Build history of the part. All positions in model axes, mm. Round coordinates to 2 decimals unless told otherwise and drop trailing zeros. Loops run counter-clockwise (first coordinate to the right, second up) from the corner with the lowest first, then second, coordinate; pieces in that order, holes last. Notation, with made-up numbers: (60, -28) - (103, -28) arc R24 ccw to (103, 10) - close; hole circle Ø10 at (7.5, -9). An arc over 180 degrees is marked (long way). Use a Markdown table: item, result.
Autodesk Inventor part; units mm, degrees
ref_plane "YZ Plane" through (0, 0, 0) normal (1, 0, 0) x (0, 1, 0)
ref_plane "XZ Plane" through (0, 0, 0) normal (0, 1, 0) x (-1, 0, 0)
ref_plane "XY Plane" through (0, 0, 0) normal (0, 0, 1) x (1, 0, 0)
sketch "Sketch1" plane through (0, 0, 0) normal (0, 0, 1) x (1, 0, 0)
  circle A0 centre (-0.2682, 25.3986) radius 2.0955
  circle A1 centre (0, 0) radius 5.2
  line L0 (-19.0905, 68.1502) -> (-19.0905, 45.2902)
  line L1 (-22.4814, 68.1502) -> (-22.4814, 45.2902)
  line L2 (28.3186, 68.1502) -> (28.3186, 45.2902)
  line L3 (31.7095, 68.1502) -> (31.7095, 45.2902)
  arc A2 (-19.0905, 68.1502) -> (-22.4814, 68.1502) centre (-20.7859, 68.1502) ccw
  arc A3 (-22.4814, 45.2902) -> (-19.0905, 45.2902) centre (-20.7859, 45.2902) ccw
  arc A4 (31.7095, 68.1502) -> (28.3186, 68.1502) centre (30.0141, 68.1502) ccw
  arc A5 (28.3186, 45.2902) -> (31.7095, 45.2902) centre (30.0141, 45.2902) ccw
  line L4 (-22.4814, 56.7202) -> (-30.1014, 56.7202)
  line L5 (-30.1014, 56.7202) -> (-30.1014, 73.8652)
  line L6 (31.7095, 56.7202) -> (39.3295, 56.7202)
  line L7 (39.3295, 56.7202) -> (39.3295, 73.8652)
  line L8 (36.1545, 77.0402) -> (-26.9264, 77.0402)
  line L9 (-30.1014, 56.7202) -> (-30.1014, 37.3371)
  line L10 (39.3295, 56.7202) -> (39.3295, 37.5617)
  line L11 (0, 0) -> (0, -10.16)
  line L12 (-2.3266, -6.5613) -> (-29.5927, 35.6134)
  line L13 (2.7652, -6.8864) -> (38.58, 35.5129)
  arc A6 (-30.1014, 37.3371) -> (-29.5927, 35.6134) centre (-26.9264, 37.3371) ccw
  arc A7 (-26.9264, 77.0402) -> (-30.1014, 73.8652) centre (-26.9264, 73.8652) ccw
  arc A8 (39.3295, 73.8652) -> (36.1545, 77.0402) centre (36.1545, 73.8652) ccw
  arc A9 (38.58, 35.5129) -> (39.3295, 37.5617) centre (36.1545, 37.5617) ccw
  arc A10 (-2.3266, -6.5613) -> (2.7652, -6.8864) centre (0.3398, -4.8376) ccw
  circle A11 centre (-8.0859, 47.3249) radius 2.1844
  circle A12 centre (17.3141, 47.3249) radius 2.1844
  point P0 (0, 0)
  point P1 (-30.1014, 77.0402)
  point P2 (-30.1014, 36.4002)
  point P3 (39.3295, 36.4002)
  dimension "d5" = 7.62
  dimension "d6" = 20.32
  dimension "d7" = 7.62
  dimension "d8" = 20.32
  dimension "d9" = 20.32
  dimension "d10" = 10.16
  dimension "d11" = 3.175
  dimension "d12" = 4.191
extrude "Extrusion1" add sketch "Sketch1" along normal blind 1.524
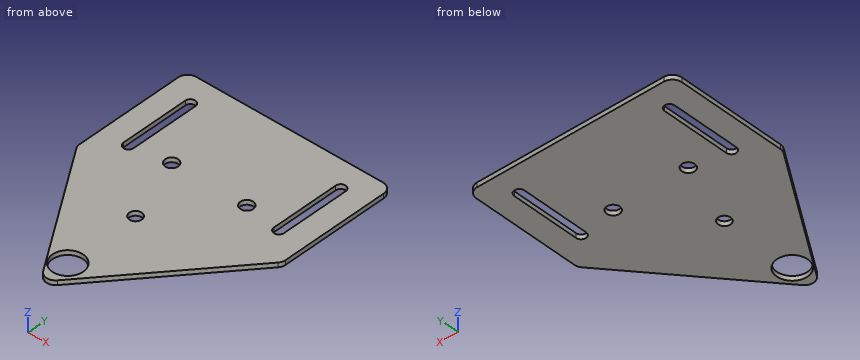
Q1. Cut at C-C, the plane x = 0. List the corners of the cut face in (y, z), plus the area to 3 significant figures.
Results found:
| item | result |
|---|---|
| outline | (-7.99, 0) - (-5.2, 0) - (-5.2, 1.52) - (-7.99, 1.52) - close; (5.2, 0) - (23.32, 0) - (23.32, 1.52) - (5.2, 1.52) - close; (27.48, 0) - (77.04, 0) - (77.04, 1.52) - (27.48, 1.52) - close |
| area | 107 mm2 |
Q2. Probe line 1 (X direction, y = 62, z = 0.9); line 2 (Y direction, x = 0, z = 0.6); line 3 (Y direction, x = 1, z = 1.2). List the from-to ranges inside material, lowest first.
Results found:
| item | result |
|---|---|
| line 1 | x = -30.1 to -22.48, -19.09 to 28.32, 31.71 to 39.33 |
| line 2 | y = -7.99 to -5.2, 5.2 to 23.32, 27.48 to 77.04 |
| line 3 | y = -7.94 to -5.1, 5.1 to 23.73, 27.07 to 77.04 |
Q3. Drop a flat-ended pin along its axis: pin 1 (4 mm diameter, centred on x = -0.27, y = 25.4, fed in from +Z). Give the stop position or say it passes through.
Results found:
| item | result |
|---|---|
| pin 1 | passes through |
Q4. Cut at D-D, the plane y = 0. List the corners of the cut face in (x, z), plus the area to 3 significant figures.
Results found:
| item | result |
|---|---|
| outline | (-6.57, 0) - (-5.2, 0) - (-5.2, 1.52) - (-6.57, 1.52) - close; (5.2, 0) - (8.58, 0) - (8.58, 1.52) - (5.2, 1.52) - close |
| area | 7.24 mm2 |
Q5. Cut at B-B, the plane z = 1.2. Count the separate pieces of the cut face and the enclosed holes in it, plus the area to 3 significant figures.
Results found:
| item | result |
|---|---|
| separate pieces | 1 |
| enclosed holes | 6 |
| area | 4,130 mm2 |
Q6. Cut at A-A, the plane y = 57. List the corners of the cut face in (x, z).
Results found:
| item | result |
|---|---|
| outline | (-30.1, 0) - (-22.48, 0) - (-22.48, 1.52) - (-30.1, 1.52) - close; (-19.09, 0) - (28.32, 0) - (28.32, 1.52) - (-19.09, 1.52) - close; (31.71, 0) - (39.33, 0) - (39.33, 1.52) - (31.71, 1.52) - close |
